Here's how the part is built. I have some questions about the finished solid (model axes, mm). Face numbers are marked on the shaded views. Round coordinates to 2 decimals unless told otherwise and drop trailing zeros. Write each loop counter-clockwise with the first axis right and the second up, starting at its lowest first coordinate (ties: lowest second). Pieces come first, ordered by that corner, then holes. Notation, with made-up numbers: (-8, 30) - (45, 30) arc R24 ccw to (45, 61) - close; hole circle Ø3 at (36, 64). An arc over 180 degrees is marked (long way). Return JSON: item names as keys, results as strings. Group by question number.
```python
from build123d import *

# Parameters (mm, degrees)
SKETCH1_R           = 7.5
BOSS_EXTRUDE1_DEPTH = 18
DOME1_FACE_RADIUS   = 7.5
DOME1_HEIGHT        = 1
FILLET1_R           = 1
SKETCH2_R           = 3.3
CUT_EXTRUDE1_DEPTH  = 6.35
SKETCH3_W           = 1.48
SKETCH3_H           = 4.164804918
BOSS_EXTRUDE2_DEPTH = 6.35


with BuildPart() as part:
    # Sketch1 → Boss-Extrude1 (new body)
    with BuildSketch(Plane(origin=(0, 0, 0), x_dir=(1, 0, 0), z_dir=(0, 1, 0))):
        with Locations(Location((0, 0, 0), (0, 0, 270))):
            Circle(SKETCH1_R)
    extrude(amount=BOSS_EXTRUDE1_DEPTH)

    # Dome1: a dome of height H over a round flat face of radius A is a cap of a sphere of radius (A * A + H * H) / (2 * H)
    dome1_r = (DOME1_FACE_RADIUS * DOME1_FACE_RADIUS + DOME1_HEIGHT * DOME1_HEIGHT) / (2 * DOME1_HEIGHT)
    dome1_base = Plane((0, 18, 0), z_dir=(0, 1, 0))
    with Locations(dome1_base.offset(DOME1_HEIGHT - dome1_r)):
        dome1_ball = Sphere(dome1_r, mode=Mode.PRIVATE)
    add(split(dome1_ball, bisect_by=dome1_base, keep=Keep.TOP, mode=Mode.PRIVATE))

    # Fillet1
    fillet1_edges = [part.edges().sort_by_distance(p)[0] for p in [
        (0, 18, -7.5),
    ]]
    fillet(fillet1_edges, radius=FILLET1_R)

    # Sketch2 → Cut-Extrude1 (cut)
    with BuildSketch(Plane.XZ):
        with Locations(Location((0, 0, 0), (0, 0, 270))):
            Circle(SKETCH2_R)
    extrude(amount=-CUT_EXTRUDE1_DEPTH, mode=Mode.SUBTRACT)

    # Sketch3 → Boss-Extrude2 (add)
    with BuildSketch(Plane.XZ.offset(-6.35)):
        with Locations((3.3, 0)):
            Rectangle(SKETCH3_W, SKETCH3_H)
    extrude(amount=BOSS_EXTRUDE2_DEPTH)


solid = part.part
```
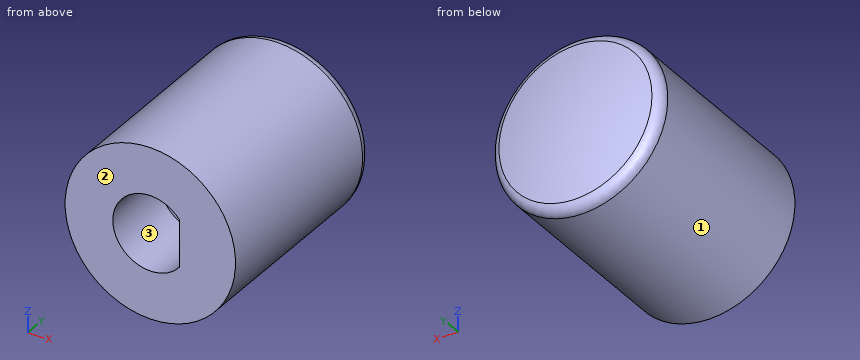
1) I need wall thicknesses on line 1 along X through (y, z) = (2, 0); line 2 along Z through (x, y) = (0, 1.5); line 3 along Z through (x, y) = (2.25, 4). Which ranges of each line are inside material? Lowest first, please.
2) Imagine slicing it at A-A (y = 2). Please give me the cut outline in (x, z), plus the area to 3 significant figures.
3) If we mould it in two halves opening along Z, with no side actions, what happens to the marked faces 1, 2 and 3? For each: released by +Z, released by -Z, zero draft, split by the parting line, or undercut.
4) Imagine slicing it at B-B (y = 11.75). Please give me the cut outline in (x, z).
5) Will these pins go through, and if not, where does the flat tip stop? pin 1 Ø1.8 at (x, z) = (0, 0.5) entering from -Y; pin 2 Ø6 at (x, y) = (5.5, 12) entering from -Z; pin 3 Ø5 at (x, y) = (-5, 8) entering from +Z.
Results found:
{
 "1": {"line 1": "x = -7.5 to -3.3, 2.56 to 7.5", "line 2": "z = -7.5 to -3.3, 3.3 to 7.5", "line 3": "z = -7.15 to -2.41, 2.41 to 7.15"},
 "2": {"outline": "circle Ø15 at (0, 0); hole (2.56, -2.08) - (2.56, 2.08) arc R3.3 ccw (long way) to start", "area": "145 mm²"},
 "3": {"face 1": "split by the parting line", "face 2": "zero draft", "face 3": "undercut"},
 "4": {"outline": "circle Ø15 at (0, 0)"},
 "5": {"pin 1": "stops at y = 6.35", "pin 2": "stops at z = -7.07", "pin 3": "stops at z = 7.07"}
}
